Geometry: final body of the model. Coordinates: model frame, mm. Face numbers are marked on the shaded views. A direction names the side the tool comes from. Give positions to 0.01 mm unless a question says otherwise; leave off trailing zeros. Write each loop counter-clockwise with the first axis right and the second up, starting at its lowest first coordinate (ties: lowest second). Pieces come first, ordered by that corner, then holes.
Q1. Mould query, pull axis Z, two halves, no side actions, for the marked faces 1, 2 and 3. Classes: +Z half, -Z half, draft (parallel to the pull), parting line (faces both ways), or undercut.
Q2. Line query: line 1 (Z direction, x = -40, y = 30); line 2 (X direction, y = 60, z = -88) (1 decimal); line 3 (X direction, y = 64.5, z = -126) (1 decimal). Output: solid intervals per line, ascending.
Q3. Pin query (flat end, axial travel): pin 1 Ø10 at (x, z) = (96.5, -92) entering from -Y; pin 2 Ø24 at (x, z) = (-101, -203.5) entering from +Y; pin 3 Ø4 at (y, z) = (84.5, -91) entering from -X; pin 4 Ø16.5 at (x, z) = (-54.5, -126) entering from +Y. Return the tip coordinate at first contact, or that it passes through.
Q4. Section C-C (z = -25.5). Return the cut outline in (x, y) (1 decimal).
Q5. Section A-A (y = 17.5). State how many separate pieces and enclosed holes the cut face has, plus the area to 3 significant figures.
Q6. Section B-B (x = 84.5). Return the cut outline in (y, z).
Q7. Reachability of the marked faces 4 and 5 from +Z, -Z, +X, -X, +Y, -Y: full face, straight path, thin tool, end or side. Return the list, or none.
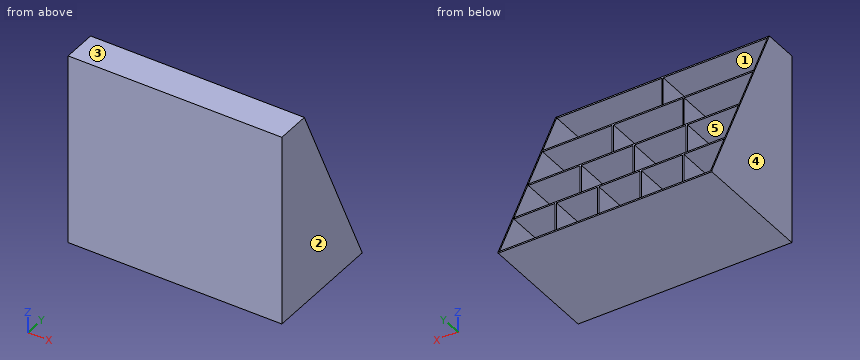
from build123d import *

# Parameters (mm, degrees)
BOSS_EXTRUDE1_DEPTH = 123.825
SKETCH3_W           = 121.44375
SKETCH3_H           = 53.578125
CUT_EXTRUDE1_DEPTH  = 38.1
SKETCH4_W           = 80.433333333
SKETCH4_H           = 53.578125
SKETCH4_W_2         = 80.433333334
CUT_EXTRUDE2_DEPTH  = 38.1
SKETCH5_W           = 59.928125
SKETCH5_H           = 53.578125
CUT_EXTRUDE3_DEPTH  = 38.1
SKETCH6_W           = 47.625
SKETCH6_H           = 53.578125
CUT_EXTRUDE4_DEPTH  = 38.1
BOSS_EXTRUDE2_DEPTH = 1.5875


with BuildPart() as part:
    # Sketch1 → Boss-Extrude1 (new, symmetric)
    with BuildSketch(Plane(origin=(0, 0, 0), x_dir=(0, 0, -1), z_dir=(1, 0, 0))):
        Polygon((0, 0), (222.25, 0), (222.25, 115.8875), (222.25, 141.2875), (220.6625, 141.2875), (220.6625, 115.8875), (165.496875, 115.8875), (165.496875, 90.4875), (110.33125, 90.4875), (110.33125, 65.0875), (55.165625, 65.0875), (55.165625, 39.6875), (0, 39.6875), (0, 14.2875), align=None)
    extrude(amount=BOSS_EXTRUDE1_DEPTH, both=True)

    # Sketch3 → Cut-Extrude1 (cut)
    with BuildSketch(Plane(origin=(0, 39.6875, 0), x_dir=(1, 0, 0), z_dir=(0, 1, 0))):
        with Locations((-61.515625, 28.3765625)):
            Rectangle(SKETCH3_W, SKETCH3_H)
        with Locations((61.515625, 28.3765625)):
            Rectangle(SKETCH3_W, SKETCH3_H)
    extrude(amount=-CUT_EXTRUDE1_DEPTH, mode=Mode.SUBTRACT)

    # Sketch4 → Cut-Extrude2 (cut)
    with BuildSketch(Plane(origin=(0, 65.0875, 0), x_dir=(1, 0, 0), z_dir=(0, 1, 0))):
        with Locations((-82.020833334, 83.5421875)):
            Rectangle(SKETCH4_W, SKETCH4_H)
        with Locations((0, 83.5421875)):
            Rectangle(SKETCH4_W_2, SKETCH4_H)
        with Locations((82.020833334, 83.5421875)):
            Rectangle(SKETCH4_W, SKETCH4_H)
    extrude(amount=-CUT_EXTRUDE2_DEPTH, mode=Mode.SUBTRACT)

    # Sketch5 → Cut-Extrude3 (cut)
    with BuildSketch(Plane(origin=(0, 90.4875, 0), x_dir=(1, 0, 0), z_dir=(0, 1, 0))):
        with Locations((-92.2734375, 138.7078125)):
            Rectangle(SKETCH5_W, SKETCH5_H)
        with Locations((-30.7578125, 138.7078125)):
            Rectangle(SKETCH5_W, SKETCH5_H)
        with Locations((30.7578125, 138.7078125)):
            Rectangle(SKETCH5_W, SKETCH5_H)
        with Locations((92.2734375, 138.7078125)):
            Rectangle(SKETCH5_W, SKETCH5_H)
    extrude(amount=-CUT_EXTRUDE3_DEPTH, mode=Mode.SUBTRACT)

    # Sketch6 → Cut-Extrude4 (cut)
    with BuildSketch(Plane(origin=(0, 115.8875, 0), x_dir=(1, 0, 0), z_dir=(0, 1, 0))):
        with Locations((-98.425, 193.8734375)):
            Rectangle(SKETCH6_W, SKETCH6_H)
        with Locations((-49.2125, 193.8734375)):
            Rectangle(SKETCH6_W, SKETCH6_H)
        with Locations((0, 193.8734375)):
            Rectangle(SKETCH6_W, SKETCH6_H)
        with Locations((49.2125, 193.8734375)):
            Rectangle(SKETCH6_W, SKETCH6_H)
        with Locations((98.425, 193.8734375)):
            Rectangle(SKETCH6_W, SKETCH6_H)
    extrude(amount=-CUT_EXTRUDE4_DEPTH, mode=Mode.SUBTRACT)

    # Sketch7 → Boss-Extrude2 (add)
    with BuildSketch(Plane(origin=(123.825, 0, 0), x_dir=(0, 0, -1), z_dir=(1, 0, 0))):
        Polygon((0, 39.6875), (220.6625, 141.2875), (220.6625, 39.6875), align=None)
    boss_extrude2 = extrude(amount=-BOSS_EXTRUDE2_DEPTH)

    # Mirror1: Boss-Extrude2 across plane
    add(boss_extrude2.mirror(Plane(origin=(0, 0, 0), x_dir=(0, 0, 1), z_dir=(1, 0, 0))))


solid = part.part
Computed:
1. face 1: undercut
1. face 2: draft
1. face 3: +Z half
2. line 1: z = -222.25 to -110.33, -56.75 to -55.17, -1.59 to 0
2. line 2: x = -123.8 to -122.2, -41.8 to -40.2, 40.2 to 41.8, 122.2 to 123.8
2. line 3: x = -123.8 to -122.2, -62.3 to -60.7, -0.8 to 0.8, 60.7 to 62.3, 122.2 to 123.8
3. pin 1: stops at y = 0
3. pin 2: stops at y = 77.79
3. pin 3: passes through
3. pin 4: stops at y = 90.49
4. outline: (-123.8, 0) - (123.8, 0) - (123.8, 51.4) - (122.2, 51.4) - (122.2, 1.6) - (0.8, 1.6) - (0.8, 39.7) - (-0.8, 39.7) - (-0.8, 1.6) - (-122.2, 1.6) - (-122.2, 51.4) - (-123.8, 51.4) - close
5. separate pieces: 1
5. enclosed holes: 2
5. area: 42,000 mm2
6. outline: (0, -222.25) - (141.29, -222.25) - (141.29, -220.66) - (77.79, -220.66) - (77.79, -167.08) - (115.89, -167.08) - (115.89, -165.5) - (52.39, -165.5) - (52.39, -111.92) - (90.49, -111.92) - (90.49, -110.33) - (26.99, -110.33) - (26.99, -56.75) - (65.09, -56.75) - (65.09, -55.17) - (1.59, -55.17) - (1.59, -1.59) - (39.69, -1.59) - (39.69, 0) - (0, 0) - close
7. face 4: +Z, -Z, -X, +Y, -Y
7. face 5: +Y
